Check sheet for the modelled part. Datum: model origin and axes. Units: mm. A direction names the side the tool comes from. Round coordinates to 2 decimals unless told otherwise and drop trailing zeros. Write each loop counter-clockwise with the first axis right and the second up, starting at its lowest first coordinate (ties: lowest second). Pieces come first, ordered by that corner, then holes.
Item 1: Cross-section at A-A on y = 0.25. Enter the section's corners in (x, z), plus the area to 3 significant figures.
Item 2: Material ranges on line 1 (Y direction, x = -5.25, z = 3.25); line 2 (X direction, y = 2, z = 5.25); line 3 (Z direction, x = -5.25, y = 2.25), recorded low to high.
Item 3: Cross-section at B-B on z = 4.5. Count the separate pieces of the cut face and the enclosed holes in it, plus the area to 3 significant figures.
Item 4: Release check for a two-part mould opening along X. For faces 1 (the flat face through (4, 0, 2)), 2 (the flat face through (10, -3, 1)), 3 (the flat face through (-5, 0, 6)) record: +X half, -X half, draft (parallel to the pull), parting line (faces both ways), or undercut.
Item 5: Go/stop test with flat-tipped pins: pin 1 Ø3 at (y, z) = (0.5, 4) entering from +X; pin 2 Ø1 at (x, z) = (8.5, 1) entering from -Y; pin 3 Ø2 at (x, y) = (-5, 0.5) entering from -Z. Record where each tip stops, or that it passes through.
Item 6: Cross-section at D-D on x = -3. Enter the section's corners in (y, z).
Item 7: Tool access check on faces 4 (the flat face through (9, -4, 1)), 5 (the flat face through (-5.574, -0.1, 6.3)), 6 (the flat face through (-3.574, -0.1, 6.3)), 7 (the flat face through (-5, 1.838, 4)), 8 (the flat face through (10, 3, 1)). Record the directions out of +Z, -Z, +X, -X, +Y, -Y that give a thin tool (end or side, any length) a straight path to the whole face; none if there is none.
from build123d import *

# Parameters (mm, degrees)
F1_DEPTH  = 2
F7_W      = 31.145259738
F7_H      = 20.1126746833
F8_DEPTH  = 25
F10_DEPTH = 4
F11_W     = 2
F11_H     = 11.6759730271
F12_DEPTH = 2
F13_R     = 3


with BuildPart() as f1:
    # F0 (on Top) → F1 (new body)
    with BuildSketch(Plane.XY):
        with BuildLine():
            ThreePointArc((8.3, 1.833030278), (8.4498520697, 0.9219544457), (8.5, 0))
            ThreePointArc((8.5, 0), (8.4498520697, -0.9219544457), (8.3, -1.833030278))
            ThreePointArc((8.3, -1.833030278), (9.0869216066, -2.3272919558), (10, -2.5))
            Line((10, -2.5), (10, 2.5))
            ThreePointArc((10, 2.5), (9.0869216066, 2.3272919558), (8.3, 1.833030278))
        make_face()
        with BuildLine():
            ThreePointArc((8.3, -1.833030278), (7.5, 0), (8.3, 1.833030278))
            ThreePointArc((8.3, 1.833030278), (7.973953815, 2.9438173442), (7.5, 4))
            Line((7.5, 4), (0, 4))
            Line((0, 4), (0, 2.5))
            ThreePointArc((0, 2.5), (1.767766953, 1.767766953), (2.5, 0))
            ThreePointArc((2.5, 0), (1.767766953, -1.767766953), (0, -2.5))
            Line((0, -2.5), (0, -4))
            Line((0, -4), (7.5, -4))
            ThreePointArc((7.5, -4), (7.973953815, -2.9438173442), (8.3, -1.833030278))
        make_face()
        with BuildLine():
            ThreePointArc((7.5, 4), (7.973953815, 2.9438173442), (8.3, 1.833030278))
            ThreePointArc((8.3, 1.833030278), (9.0869216066, 2.3272919558), (10, 2.5))
            Line((10, 2.5), (10, 4))
            Line((10, 4), (7.5, 4))
        make_face()
        with BuildLine():
            ThreePointArc((10, -2.5), (9.0869216066, -2.3272919558), (8.3, -1.833030278))
            ThreePointArc((8.3, -1.833030278), (7.973953815, -2.9438173442), (7.5, -4))
            Line((7.5, -4), (10, -4))
            Line((10, -4), (10, -2.5))
        make_face()
        with BuildLine():
            Line((0, 4), (7.5, 4))
            ThreePointArc((7.5, 4), (-8.5, 0), (7.5, -4))
            Line((7.5, -4), (0, -4))
            Line((0, -4), (0, -2.5))
            ThreePointArc((0, -2.5), (-2.5, 0), (0, 2.5))
            Line((0, 2.5), (0, 4))
        make_face()
        with BuildLine():
            ThreePointArc((12.5, 0), (11.767766953, 1.767766953), (10, 2.5))
            Line((10, 2.5), (10, -2.5))
            ThreePointArc((10, -2.5), (11.767766953, -1.767766953), (12.5, 0))
        make_face()
        with BuildLine():
            ThreePointArc((8.3, -1.833030278), (8.4498520697, -0.9219544457), (8.5, 0))
            ThreePointArc((8.5, 0), (8.4498520697, 0.9219544457), (8.3, 1.833030278))
            ThreePointArc((8.3, 1.833030278), (7.5, 0), (8.3, -1.833030278))
        make_face()
        with BuildLine():
            ThreePointArc((2.5, 0), (1.767766953, 1.767766953), (0, 2.5))
            Line((0, 2.5), (0, -2.5))
            ThreePointArc((0, -2.5), (1.767766953, -1.767766953), (2.5, 0))
        make_face()
        with BuildLine():
            Line((0, -2.5), (0, 2.5))
            ThreePointArc((0, 2.5), (-2.5, 0), (0, -2.5))
        make_face()
    extrude(amount=F1_DEPTH)

    # F6: sweep along a path in F5
    with BuildLine(Plane(origin=(0, 0, 0), x_dir=(-1, 0, 0), z_dir=(0, 1, 0))) as f6_path:
        ThreePointArc((0, 0), (-5, 6.024653635), (-10, 0))
    # F3 (on line) → F6 (sweep)
    with BuildSketch(Plane.YZ.offset(5)):
        with BuildLine():
            ThreePointArc((0, 3.524653635), (1.767766953, 4.256886682), (2.5, 6.024653635))
            ThreePointArc((2.5, 6.024653635), (-1.767766953, 7.792420588), (0, 3.524653635))
        make_face()
    sweep(path=f6_path.line)

    # F7 (on Top) → F8 (cut)
    with BuildSketch(Plane.XY):
        Rectangle(F7_W, F7_H)
    extrude(amount=-F8_DEPTH, mode=Mode.SUBTRACT)

    # F9 (on face) → F10 (join)
    with BuildSketch(Plane.XY.offset(2)):
        Polygon((-3.5739342159, 1.8379865136), (-3.5739342159, 2.9988868824), (-3.5739342159, 5.8379865136), (-5.5739342159, 5.8379865136), (-5.5739342159, 1.8379865136), align=None)
        Polygon((-3.5739342159, -5.8379865136), (-3.5739342159, -2.9988868824), (-3.5739342159, -1.8379865136), (-5.5739342159, -1.8379865136), (-5.5739342159, -5.8379865136), align=None)
    extrude(amount=F10_DEPTH)

    # F11 (on face) → F12 (join)
    with BuildSketch(Plane.XY.offset(6)):
        with Locations((-4.5739342159, 0)):
            Rectangle(F11_W, F11_H)
    extrude(amount=F12_DEPTH)

    # F13
    f13_edges = [f1.edges().sort_by_distance(p)[0] for p in [
        (-4.573934, -5.837987, 8),
        (-4.573934, 5.837987, 8),
    ]]
    fillet(f13_edges, radius=F13_R)


solid = f1.part
Response values:
1. outline: (-8.5, 0) - (12.52, 0) arc R7.57 ccw to (-2.5, 2) - (-8.5, 2) - close; (-5.57, 6) - (-3.57, 6) - (-3.57, 8) - (-5.57, 8) - close; hole (2.63, 2) - (7.37, 2) arc R2.6 ccw to start
1. area: 115 mm2
2. line 1: y = -5.84 to -1.84, 1.84 to 5.84
2. line 2: x = -5.57 to -3.57, 0.02 to 9.98
2. line 3: z = 0 to 8
3. separate pieces: 3
3. enclosed holes: 0
3. area: 73.0 mm2
4. face 1: undercut
4. face 2: +X half
4. face 3: draft
5. pin 1: stops at x = 12.41
5. pin 2: stops at y = -4
5. pin 3: stops at z = 0
6. outline: (-7.95, 0) - (7.95, 0) - (7.95, 2) - (-7.95, 2) - close
7. face 4: +Z, -Z, +X, -Y
7. face 5: +Z, -X, +Y, -Y
7. face 6: +Z, +Y, -Y
7. face 7: -X
7. face 8: +Z, -Z, +X, +Y
